The listing builds one solid part. Answer for the finished solid, in the listing's coordinates (mm). A direction names the side the tool comes from. Coordinates: 2 decimals unless noted, no trailing zeros. Order: outer loops, then holes, each group sorted by start corner. A loop starts at its lowest first (then second) coordinate and runs counter-clockwise, first axis right, second up. Notation, with made-up numbers: (40.25, 34) -> (51.25, 34) arc R14 cw to (51.25, 59) -> close; hole circle Ø10 at (2.5, 8.5). An arc over 180 degrees is marked (long way). Write each question's results on one line, items separated by ' | '. Start each with the question number.
(1) A tool of negligible diameter and unlimited length cuts with its end or side. For faces 1 (the face through (-14.188, 1.232, 30.607)), 2 (the face through (-14, 4, 34.682)), 3 (the face through (-57, 4, -36.318)), 4 (the face through (-12.874, 9, -33)), 5 (the face through (-9.874, 11, 0)), from which of +Z, -Z, +X, -X, +Y, -Y can it reach the whole face along a straight path? Write none if from no direction.
(2) Straight lines are drawn through the part: L1, parallel to X at y = 5.5, z = -16; L2, parallel to Z at x = -55.5, y = 10.25; L3, parallel to Y at x = -55, z = 20.5. For each, find the intervals that lie inside material, in ascending order.
(3) The part is cut by section B-B, the plane y = 10.25. Give the vertices of the cut face in (x, z), then the cut area to 3 significant figures.
(4) The part is cut by section A-A, the plane y = 16.75. Give the vertices of the cut face in (x, z).
(5) The part is cut by section D-D, the plane y = 5.25. Give the vertices of the cut face in (x, z), then the cut area to 3 significant figures.
(6) Determine the mould class of faces 6 (the face through (-58.874, 9, 0)), 7 (the face through (-52.874, 5, -33)), 8 (the face through (-18.374, 5, 31)) for opening direction X: +X half, -X half, draft (parallel to the pull), parting line (faces both ways), or undercut.
(7) The part is cut by section C-C, the plane z = -12.5. Give the vertices of the cut face in (x, y).
(8) Given pin 1 (3 mm diameter, centred on x = -36.5, z = 27.5, fed in from -Y); pin 2 (3 mm diameter, centred on x = -55.37, z = -33.32, fed in from -Y); pin 3 (1.2 mm diameter, centred on y = 4, z = 30, fed in from +X), each flat-ended and moving along its own axis, determine where each tip first touches the part or whether it passes through.
```python
from build123d import *

# Parameters (mm, degrees)
SKETCH1_W           = 51.5
SKETCH1_H           = 73
BOSS_EXTRUDE1_DEPTH = 22
CUT_EXTRUDE1_DEPTH  = 18
SKETCH4_R           = 2
CUT_EXTRUDE2_DEPTH  = 16
SKETCH7_W           = 7
SKETCH7_H           = 4
CUT_EXTRUDE3_DEPTH  = 8.5
SKETCH9_W           = 7
SKETCH9_H           = 4
CUT_EXTRUDE4_DEPTH  = 8.5


with BuildPart() as part:
    # Sketch1 → Boss-Extrude1 (new body)
    with BuildSketch(Plane(origin=(0, 0, 0), x_dir=(1, 0, 0), z_dir=(0, 1, 0))):
        with Locations((-35.624481527, 0.818123821)):
            Rectangle(SKETCH1_W, SKETCH1_H)
    extrude(amount=BOSS_EXTRUDE1_DEPTH)

    # Sketch2 → Cut-Extrude1 (cut)
    with BuildSketch(Plane.XZ):
        Polygon((-58.374481527, 27.681876179), (-58.874481527, 27.681876179), (-58.874481527, -29.318123821), (-52.374481527, -29.318123821), (-52.374481527, -37.318123821), (-12.874481527, -37.318123821), (-12.874481527, -29.318123821), (-11.875874941, -29.318123821), (-11.875874941, 27.681876179), (-18.874481527, 27.681876179), (-18.874481527, 35.681876179), (-54.374481527, 35.681876179), (-58.374481527, 35.681876179), align=None)
    extrude(amount=-CUT_EXTRUDE1_DEPTH, mode=Mode.SUBTRACT)

    # Sketch4 → Cut-Extrude2 (cut)
    with BuildSketch(Plane.XZ):
        with Locations(Location((-15.874481527, 31.681876179, 0), (0, 0, 270))):
            Circle(SKETCH4_R)
        with Locations(Location((-55.374481527, -33.318123821, 0), (0, 0, 270))):
            Circle(SKETCH4_R)
    extrude(amount=-CUT_EXTRUDE2_DEPTH, mode=Mode.SUBTRACT)

    # Sketch7 → Cut-Extrude3 (cut)
    with BuildSketch(Plane.ZY.offset(61.374481527)):
        with Locations((-32.818123821, 4.5)):
            Rectangle(SKETCH7_W, SKETCH7_H)
    extrude(amount=-CUT_EXTRUDE3_DEPTH, mode=Mode.SUBTRACT)

    # Sketch9 → Cut-Extrude4 (cut)
    with BuildSketch(Plane(origin=(-9.874481527, 0, 0), x_dir=(0, 0, -1), z_dir=(1, 0, 0))):
        with Locations((-31.181876179, 4.5)):
            Rectangle(SKETCH9_W, SKETCH9_H)
    extrude(amount=-CUT_EXTRUDE4_DEPTH, mode=Mode.SUBTRACT)


solid = part.part
```
Established:
1) face 1: -Y | face 2: +X | face 3: -X | face 4: -Z, -Y | face 5: +Z, -Z, +X, +Y, -Y
2) L1: x = -61.37 to -58.87, -11.88 to -9.87 | L2: z = -37.32 to -35.31, -31.32 to -29.32 | L3: y = 18 to 22
3) outline: (-61.37, -37.32) -> (-52.37, -37.32) -> (-52.37, -29.32) -> (-58.87, -29.32) -> (-58.87, 27.68) -> (-58.37, 27.68) -> (-58.37, 35.68) -> (-61.37, 35.68) -> close; (-18.87, 27.68) -> (-11.88, 27.68) -> (-11.88, -29.32) -> (-12.87, -29.32) -> (-12.87, -37.32) -> (-9.87, -37.32) -> (-9.87, 35.68) -> (-18.87, 35.68) -> close; hole circle Ø4 at (-55.37, -33.32); hole circle Ø4 at (-15.87, 31.68) | area: 423 mm^2
4) outline: (-61.37, -37.32) -> (-52.37, -37.32) -> (-52.37, -29.32) -> (-58.87, -29.32) -> (-58.87, 27.68) -> (-58.37, 27.68) -> (-58.37, 35.68) -> (-61.37, 35.68) -> close; (-18.87, 27.68) -> (-11.88, 27.68) -> (-11.88, -29.32) -> (-12.87, -29.32) -> (-12.87, -37.32) -> (-9.87, -37.32) -> (-9.87, 35.68) -> (-18.87, 35.68) -> close
5) outline: (-61.37, -37.32) -> (-52.37, -37.32) -> (-52.37, -29.32) -> (-52.87, -29.32) -> (-52.87, -36.32) -> (-61.37, -36.32) -> close; (-61.37, -29.32) -> (-58.87, -29.32) -> (-58.87, 27.68) -> (-58.37, 27.68) -> (-58.37, 35.68) -> (-61.37, 35.68) -> close; (-18.87, 27.68) -> (-18.37, 27.68) -> (-18.37, 34.68) -> (-9.87, 34.68) -> (-9.87, 35.68) -> (-18.87, 35.68) -> close; (-12.87, -37.32) -> (-9.87, -37.32) -> (-9.87, 27.68) -> (-11.88, 27.68) -> (-11.88, -29.32) -> (-12.87, -29.32) -> close | area: 330 mm^2
6) face 6: undercut | face 7: -X half | face 8: +X half
7) outline: (-61.37, 0) -> (-58.87, 0) -> (-58.87, 18) -> (-11.88, 18) -> (-11.88, 0) -> (-9.87, 0) -> (-9.87, 22) -> (-61.37, 22) -> close
8) pin 1: stops at y = 18 | pin 2: stops at y = 16 | pin 3: stops at x = -18.37
